Verification items for the finished model (mm, model axes). Face numbers are marked on the shaded views. A direction names the side the tool comes from. Give positions to 0.01 mm unless a question says otherwise; leave off trailing zeros. Loops run counter-clockwise (first coordinate to the right, second up) from the corner with the lowest first, then second, coordinate; pieces in that order, holes last. Notation, with made-up numbers: M 74,87 L 95,87 A16 cw 95,113 Z; hole C 61,-28.75 d5. An arc over 180 degrees is marked long. Use a Markdown table: item, result.
from build123d import *

# Parameters (mm, degrees)
SKETCH1_W         = 50
SKETCH1_H         = 50
SKETCH1_R         = 1.5
SUPPORT_DEPTH     = 8
SOUTH_START       = 25
SKETCH2_W         = 20
SKETCH2_H         = 5
SOUTH_DOWEL_DEPTH = 4
WEST_START        = 25
SKETCH3_W         = 20
SKETCH3_H         = 5
WEST_DOWEL_DEPTH  = 4


with BuildPart() as part:
    # Sketch1 → Support (new body)
    with BuildSketch(Plane(origin=(0, 0, 0), x_dir=(1, 0, 0), z_dir=(0, 1, 0))):
        Rectangle(SKETCH1_W, SKETCH1_H)
        with Locations(Location((-21, -21, 0), (0, 0, 270))):
            Circle(SKETCH1_R, mode=Mode.SUBTRACT)
        with Locations(Location((21, -21, 0), (0, 0, 270))):
            Circle(SKETCH1_R, mode=Mode.SUBTRACT)
        with BuildLine():
            Line((-13.031373033, 17.5), (17.5, 17.5))
            Line((17.5, 17.5), (17.5, -17.5))
            Line((17.5, -17.5), (-17.5, -17.5))
            Line((-17.5, -17.5), (-17.5, 13.031373033))
            ThreePointArc((-17.5, 13.031373033), (-20, 14.354248689), (-21, 17))
            Line((-21, 17), (-22.130136986, 20.01369863))
            ThreePointArc((-22.130136986, 20.01369863), (-22.060660172, 22.060660172), (-20.01369863, 22.130136986))
            Line((-20.01369863, 22.130136986), (-17, 21))
            ThreePointArc((-17, 21), (-14.354248689, 20), (-13.031373033, 17.5))
        make_face(mode=Mode.SUBTRACT)
        with Locations(Location((21, 21, 0), (0, 0, 270))):
            Circle(SKETCH1_R, mode=Mode.SUBTRACT)
    extrude(amount=SUPPORT_DEPTH)

    # Sketch2 → South Dowel (add)
    with BuildSketch(Plane.XY.offset(SOUTH_START)):
        with Locations((0, 4)):
            Rectangle(SKETCH2_W, SKETCH2_H)
    extrude(amount=SOUTH_DOWEL_DEPTH)

    # Sketch3 → West Dowel (add)
    with BuildSketch(Plane(origin=(0, 0, 0), x_dir=(0, 0, -1), z_dir=(1, 0, 0)).offset(WEST_START)):
        with Locations((0, 4)):
            Rectangle(SKETCH3_W, SKETCH3_H)
    extrude(amount=WEST_DOWEL_DEPTH)


solid = part.part
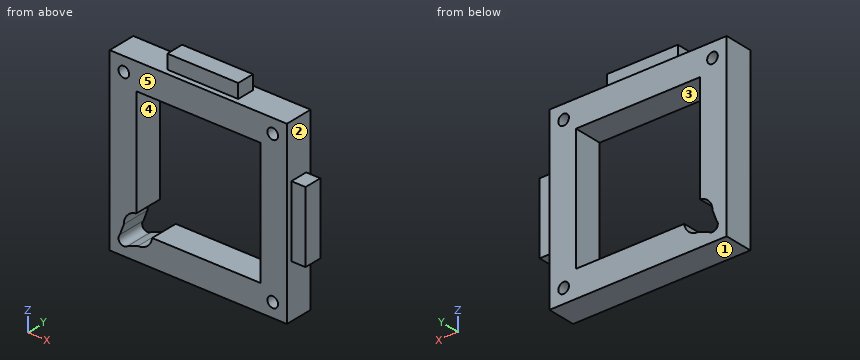
(1) Cross-section at A-A on x = 21. Record the cut outline in (y, z), then the cut area to 3 significant figures.
Results below:
| item | result |
|---|---|
| outline | M 0,-25 L 8,-25 L 8,-22.5 L 0,-22.5 Z; M 0,-19.5 L 8,-19.5 L 8,19.5 L 0,19.5 Z; M 0,22.5 L 8,22.5 L 8,25 L 0,25 Z |
| area | 352 mm^2 |
(2) Gauge pin test, flat ends, axial feed: P1, Ø3, axis at x = 27, y = 3.5, coming from the -Z side; P2, Ø3, axis at y = 7, z = -15, coming from the +X side; P3, Ø2, axis at x = 26.5, z = -3, coming from the +Y side. Record the tip position at first contact, or that the pin passes through.
Results below:
| item | result |
|---|---|
| P1 | z = -10 |
| P2 | x = 25 |
| P3 | y = 6.5 |
(3) Cross-section at C-C on y = 3. Record the cut outline in (x, z), then the cut area to 3 significant figures.
Results below:
| item | result |
|---|---|
| outline | M -25,-25 L 25,-25 L 25,-10 L 29,-10 L 29,10 L 25,10 L 25,25 L 10,25 L 10,29 L -10,29 L -10,25 L -25,25 Z; hole C -21,21 d3; hole M -22.13,-20.01 A1.5 ccw -20.01,-22.13 L -17,-21 A4 ccw -13.03,-17.5 L 17.5,-17.5 L 17.5,17.5 L -17.5,17.5 L -17.5,-13.03 A4 ccw -21,-17 Z; hole C 21,-21 d3; hole C 21,21 d3 |
| area | 1,370 mm^2 |
(4) Set-up check for the marked faces 4 and 5: record each of +Z, -Z, +X, -X, +Y, -Y from which the full face is reachable in a straight line by a thin tool's end or side.
Results below:
| item | result |
|---|---|
| face 4 | +Y, -Y |
| face 5 | +Z, -Z, +X, -X, -Y |
(5) Draft check along Z on the marked faces 1, 2 and 3. Enter one of: +Z half, -Z half, draft (parallel to the pull), parting line (faces both ways), or undercut.
Results below:
| item | result |
|---|---|
| face 1 | -Z half |
| face 2 | draft |
| face 3 | undercut |
(6) Material ranges on line 1 (X direction, y = 4.25, z = 21); line 2 (X direction, y = 5.5, z = -3); line 3 (Z direction, x = -10, y = 0.5), recorded low to high.
Results below:
| item | result |
|---|---|
| line 1 | -25 to -22.5, -19.5 to 19.5, 22.5 to 25 |
| line 2 | -25 to -17.5, 17.5 to 29 |
| line 3 | -25 to -17.5, 17.5 to 25 |
(7) Cross-section at D-D on x = 12.5. Record the cut outline in (y, z).
Results below:
| item | result |
|---|---|
| outline | M 0,-25 L 8,-25 L 8,-17.5 L 0,-17.5 Z; M 0,17.5 L 8,17.5 L 8,25 L 0,25 Z |
(8) Cross-section at B-B on z = -11.5. Record the cut outline in (x, y).
Results below:
| item | result |
|---|---|
| outline | M -25,0 L -17.5,0 L -17.5,8 L -25,8 Z; M 17.5,0 L 25,0 L 25,8 L 17.5,8 Z |
